Source: CAD feature listing. Evaluate the final solid. Frame: model axes, mm. Face numbers are marked on the shaded views. Round coordinates to 2 decimals unless told otherwise and drop trailing zeros. Loops run counter-clockwise (first coordinate to the right, second up) from the corner with the lowest first, then second, coordinate; pieces in that order, holes last. Notation, with made-up numbers: M -25.5,66 L 28.5,66 A19 ccw 28.5,88 Z; hole C 43.25,67.5 d4. An arc over 180 degrees is marked long. Write each question's results on one line, items separated by ' | '. Start each with the question number.
1. Contact query for flat-ended pins moving along their axis: pin 1 Ø1.5 at (y, z) = (-0.5, -1.5) entering from -X; pin 2 Ø0.6 at (x, z) = (0, 0) entering from -Y. Output: stop coordinate, or through.
2. Section A-A on x = 0. Output: boundary loops of the cut face in (y, z), and give its area (3 significant figures).
3. Ray query, line 1 (Y direction, x = -0.7, z = -0.2); line 2 (Z direction, x = 0.45, y = -6.5); line 3 (Z direction, x = 1.7, y = 1.5). Return the intervals inside material, ascending.
4. Draft query along Z for the marked faces 1, 2 and 3. Return one class per face: released by +Z, released by -Z, zero draft, split by the parting line, or undercut.
5. Section B-B on z = 0. Output: boundary loops of the cut face in (x, y) (3 decimals).
6. Section C-C on y = -2. Output: boundary loops of the cut face in (x, z).
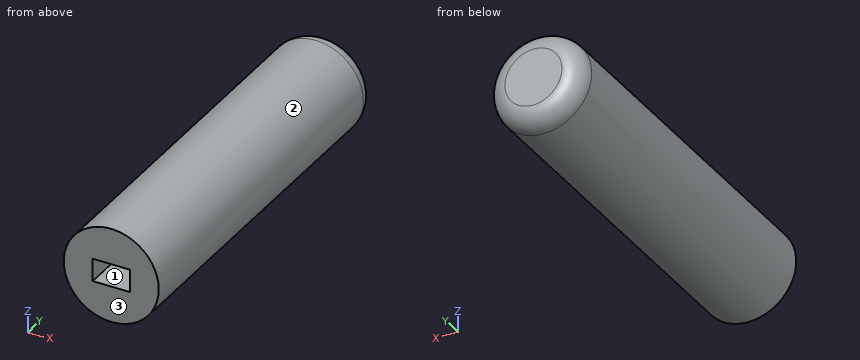
from build123d import *

# Parameters (mm, degrees)
SKETCH2_R           = 2.5
SKETCH2_W           = 1.95
SKETCH2_H           = 1.2
BOSS_EXTRUDE1_DEPTH = 10
FILLET1_R           = 1
SKETCH3_W           = 1.95
SKETCH3_H           = 1.2
BOSS_EXTRUDE5_DEPTH = 16


with BuildPart() as part:
    # Sketch2 → Boss-Extrude1 (new body, symmetric)
    with BuildSketch(Plane(origin=(0, 0, 0), x_dir=(1, 0, 0), z_dir=(0, 1, 0))):
        Circle(SKETCH2_R)
        Rectangle(SKETCH2_W, SKETCH2_H, mode=Mode.SUBTRACT)
    extrude(amount=BOSS_EXTRUDE1_DEPTH, both=True)

    # Fillet1
    fillet1_edges = [part.edges().sort_by_distance(p)[0] for p in [
        (-2.5, 10, 0),
    ]]
    fillet(fillet1_edges, radius=FILLET1_R)

    # Sketch3 → Boss-Extrude5 (add)
    with BuildSketch(Plane(origin=(0, 10, 0), x_dir=(1, 0, 0), z_dir=(0, 1, 0))):
        Rectangle(SKETCH3_W, SKETCH3_H)
    extrude(amount=-BOSS_EXTRUDE5_DEPTH)


solid = part.part
Taken from the geometry:
1) pin 1: x = -2.38 | pin 2: y = -6
2) outline: M -10,-2.5 L 9,-2.5 A1 ccw 10,-1.5 L 10,1.5 A1 ccw 9,2.5 L -10,2.5 L -10,0.6 L -6,0.6 L -6,-0.6 L -10,-0.6 Z | area: 94.8 mm^2
3) line 1: -6 to 10 | line 2: -2.46 to -0.6, 0.6 to 2.46 | line 3: -1.83 to 1.83
4) face 1: undercut | face 2: split by the parting line | face 3: zero draft
5) outline: M -2.5,-10 L -0.975,-10 L -0.975,-6 L 0.975,-6 L 0.975,-10 L 2.5,-10 L 2.5,9 A1 ccw 1.5,10 L -1.5,10 A1 ccw -2.5,9 Z
6) outline: C 0,0 d5
